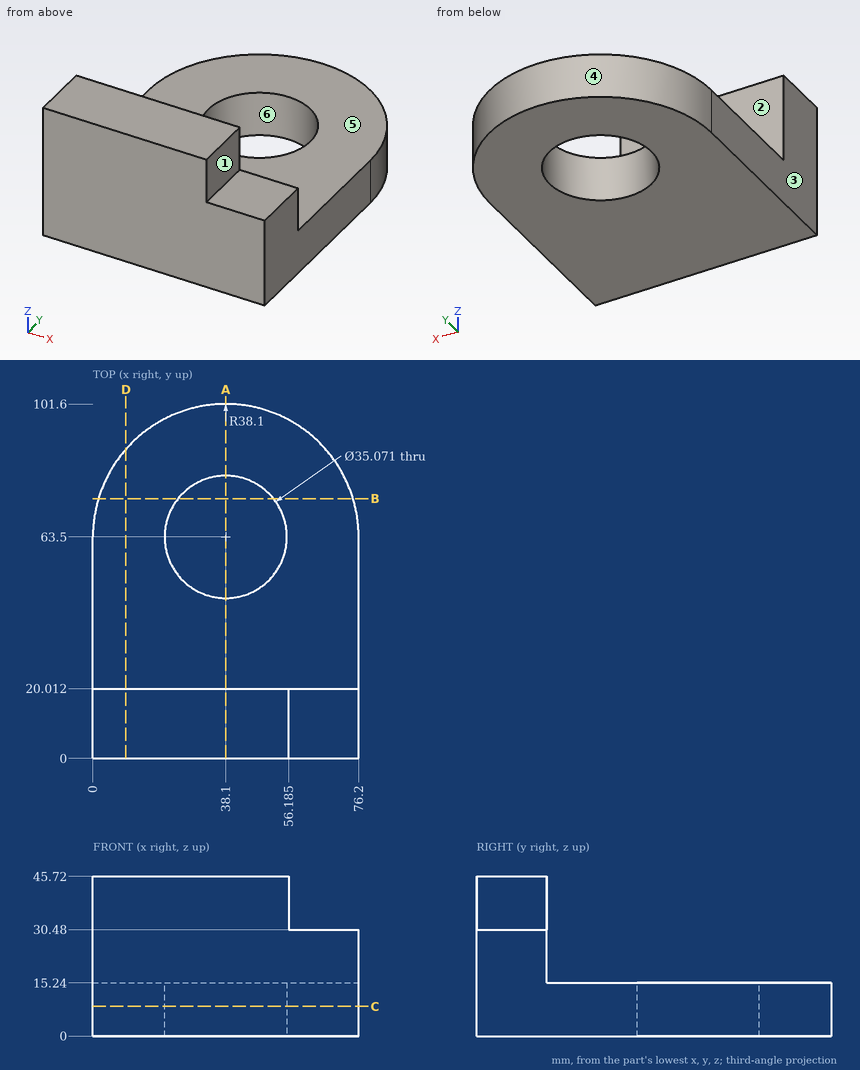
Geometry check sheet. Reference: drawing and pictorial views, mm from the part's lowest x, y, z. A direction names the side the tool comes from. Coordinates: 2 decimals unless noted, no trailing zeros. Loops run counter-clockwise (first coordinate to the right, second up) from the corner with the lowest first, then second, coordinate; pieces in that order, holes last. Notation, with made-up numbers: (50.25, 60.25) -> (99.25, 60.25) arc R23 ccw to (99.25, 70.25) -> close; hole circle Ø9 at (30.25, 11). An arc over 180 degrees is marked (long way). Write item = value, one per line. Start each with the question number.
1. Tool access check on the marked faces 1, 2 and 3. Record the directions out of +Z, -Z, +X, -X, +Y, -Y that give a thin tool (end or side, any length) a straight path to the whole face; none if there is none.
2. Material ranges on line 1 (Y direction, x = 38.1, z = 8.75) (1 decimal); line 2 (X direction, y = 63, z = 4); line 3 (Z direction, x = 65, y = 47), recorded low to high.
3. Section check D-D on x = 9.5. Record the cut outline in (y, z), then the cut area to 3 significant figures.
4. Section check B-B on y = 74.5. Record the cut outline in (x, z).
5. Draft check along X on the marked faces 4, 5 and 6. Enter one of: released by +X, released by -X, zero draft, split by the parting line, or undercut.
6. Depth check by flat-ended pin: P1, Ø15, axis at x = 43.5, z = 30, coming from the +Y side; P2, Ø3, axis at x = 46.5, z = 11.5, coming from the +Y side; P3, Ø23, axis at x = 35, y = 75, coming from the +Z side. Enter the tip coordinate at first touch or a pass-through.
7. Section check C-C on z = 8.5. Record the cut outline in (x, y) (1 decimal), then the cut area to 3 significant figures.
8. Section check A-A on x = 38.1. Record the cut outline in (y, z) (1 decimal).
Responses:
q1.face_1 = +Z, +X, +Y, -Y
q1.face_2 = +Z, +X, -X, +Y
q1.face_3 = +Z, -Z, -X, +Y, -Y
q2.line_1 = 0 to 46, 81 to 101.6
q2.line_2 = 0 to 20.57, 55.63 to 76.2
q2.line_3 = 0 to 15.24
q3.outline = (0, 0) -> (88.67, 0) -> (88.67, 15.24) -> (20.01, 15.24) -> (20.01, 45.72) -> (0, 45.72) -> close
q3.area = 1,960 mm2
q4.outline = (1.62, 0) -> (24.44, 0) -> (24.44, 15.24) -> (1.62, 15.24) -> close; (51.76, 0) -> (74.58, 0) -> (74.58, 15.24) -> (51.76, 15.24) -> close
q5.face_4 = split by the parting line
q5.face_5 = zero draft
q5.face_6 = undercut
q6.P1 = 20.01
q6.P2 = 100.97
q6.P3 = 15.24
q7.outline = (0, 0) -> (76.2, 0) -> (76.2, 63.5) arc R38.1 ccw to (0, 63.5) -> close; hole circle Ø35.1 at (38.1, 63.5)
q7.area = 6,150 mm2
q8.outline = (0, 0) -> (46, 0) -> (46, 15.2) -> (20, 15.2) -> (20, 45.7) -> (0, 45.7) -> close; (81, 0) -> (101.6, 0) -> (101.6, 15.2) -> (81, 15.2) -> close
